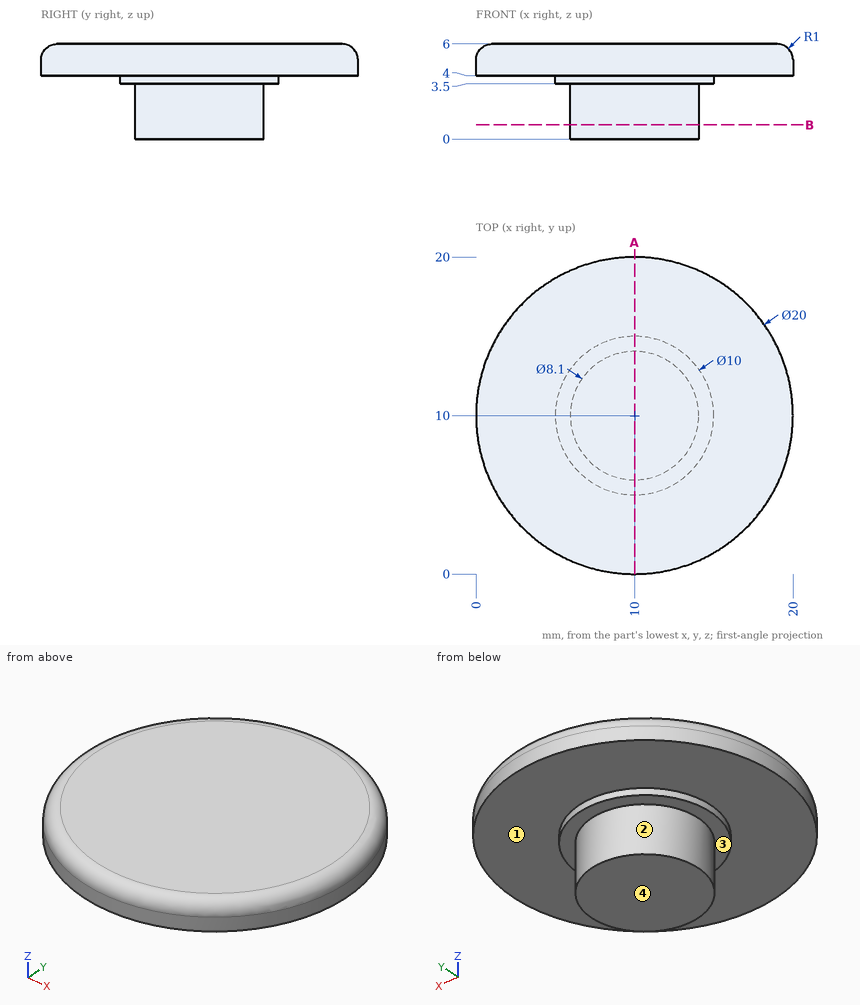
For this review, use the dimensioned drawing (mm, ordinates from the lowest corner) and the shaded views. A direction names the side the tool comes from. Coordinates: 2 decimals unless noted, no trailing zeros. Loops run counter-clockwise (first coordinate to the right, second up) from the corner with the lowest first, then second, coordinate; pieces in that order, holes last. Notation, with made-up numbers: (64.25, 2) - (84.25, 2) arc R20 ccw to (84.25, 19) - close; hole circle Ø6 at (14.25, 17.5). An arc over 180 degrees is marked (long way). Use one line per item in the form item = value. Start each with the question number.
1) For pin 1 (1.5 mm diameter, centred on y = 13, z = 5, fed in from -X); pin 2 (12 mm diameter, centred on x = 12.5, y = 12, fed in from -Z); pin 3 (1 mm diameter, centred on x = 9, z = 1, fed in from +Y); pin 4 (3 mm diameter, centred on x = 13.5, z = 5, fed in from +Y), all flat-tipped, find the tip position at first contact; note any pin that passes through.
2) For the marked faces 3 and 4, list the 3-axis set-ups (+Z, -Z, +X, -X, +Y, -Y) from which the entire face can be reached by the end or side of a thin tool; tool diameter is ignored.
3) Take a section at A-A (x = 10). State the section outline as (y, z) points.
4) Take a section at B-B (z = 0.9). State the section outline as (x, y) points, plus the area to 3 significant figures.
5) Draft analysis for pull direction X (two halves, no side actions). For the marked faces 1 and 2, state which applies: released by +X, released by -X, zero draft, split by the parting line, or undercut.
6) To check wall thickness, follow probe 1 along Z at (x, y) = (4.5, 12); probe 2 along Z at (x, y) = (13.25, 7.5); probe 3 along X at (y, z) = (12.5, 5.2). State the ranges of each line that lie inside material, in increasing order. Write a range as from..to.
From the geometry:
q1.pin_1 = 0.26
q1.pin_2 = 0
q1.pin_3 = 14.02
q1.pin_4 = 19.8
q2.face_3 = -Z
q2.face_4 = -Z, +X, -X, +Y, -Y
q3.outline = (0, 4) - (5, 4) - (5, 3.5) - (5.95, 3.5) - (5.95, 0) - (14.05, 0) - (14.05, 3.5) - (15, 3.5) - (15, 4) - (20, 4) - (20, 5) arc R1 ccw to (19, 6) - (1, 6) arc R1 ccw to (0, 5) - close
q4.outline = circle Ø8.1 at (10, 10)
q4.area = 51.5 mm2
q5.face_1 = zero draft
q5.face_2 = split by the parting line
q6.probe_1 = 4..6
q6.probe_2 = 3.5..6
q6.probe_3 = 0.34..19.66
